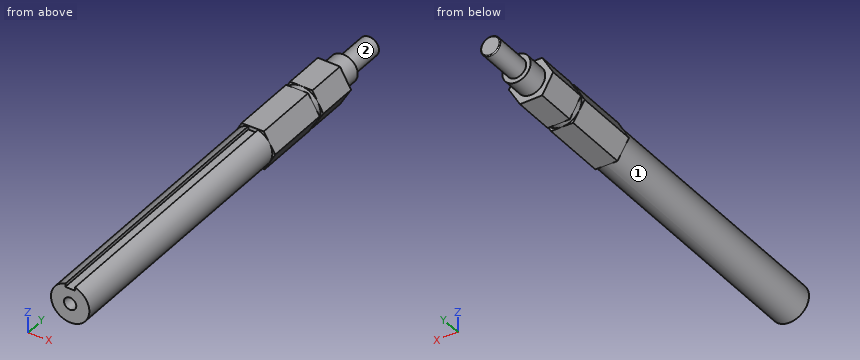
Autodesk Inventor part; units mm, degrees
ref_plane "YZ Plane" through (0, 0, 0) normal (1, 0, 0) x (0, 1, 0)
ref_plane "XZ Plane" through (0, 0, 0) normal (0, 1, 0) x (-1, 0, 0)
ref_plane "XY Plane" through (0, 0, 0) normal (0, 0, 1) x (1, 0, 0)
sketch "Sketch1" plane through (0, 0, 0) normal (0, 1, 0) x (-1, 0, 0)
  circle A0 centre (0, 0) radius 6.35
  dimension "d0" = 12.7
extrude "Extrusion1" add sketch "Sketch1" along normal mid plane 88.9
sketch "Sketch2" plane through (0, 44.45, 0) normal (0, 1, 0) x (1, 0, 0)
  circle A0 centre (0, 0) radius 6.35
  line L0 (3.8092, 6.2652) -> (7.3305, -0.1662)
  line L1 (7.3305, -0.1662) -> (3.5213, -6.4315)
  line L2 (3.5213, -6.4315) -> (-3.8092, -6.2652)
  line L3 (-3.8092, -6.2652) -> (-7.3305, 0.1662)
  line L4 (-7.3305, 0.1662) -> (-3.5213, 6.4315)
  line L5 (-3.5213, 6.4315) -> (3.8092, 6.2652)
  dimension "d4" = 12.7
extrude "Extrusion2" add sketch "Sketch2" along normal blind 21.59
sketch "Sketch3" plane through (0, 66.04, 0) normal (0, 1, 0) x (1, 0, 0)
  circle A0 centre (0, 0) radius 6.35
  dimension "d7" = 12.7
extrude "Extrusion3" add sketch "Sketch3" along normal blind 1.778
sketch "Sketch4" plane through (0, 67.818, 0) normal (0, 1, 0) x (1, 0, 0)
  circle A0 centre (0, 0) radius 6.35
  line L0 (7.3323, 0) -> (3.6662, -6.35)
  line L1 (3.6662, -6.35) -> (-3.6662, -6.35)
  line L2 (-3.6662, -6.35) -> (-7.3323, 0)
  line L3 (-7.3323, 0) -> (-3.6662, 6.35)
  line L4 (-3.6662, 6.35) -> (3.6662, 6.35)
  line L5 (3.6662, 6.35) -> (7.3323, 0)
  dimension "d10" = 12.7
extrude "Extrusion4" add sketch "Sketch4" along normal blind 13.462
sketch "Sketch5" plane through (0, 81.28, 0) normal (0, 1, 0) x (1, 0, 0)
  circle A0 centre (0, 0) radius 4.699
  dimension "d13" = 9.398
extrude "Extrusion5" add sketch "Sketch5" along normal blind 7.112
sketch "Sketch6" plane through (0, 88.392, 0) normal (0, 1, 0) x (1, 0, 0)
  circle A0 centre (0, 0) radius 4.699
  circle A1 centre (0, 0) radius 3.2258
  dimension "d16" = 6.4516
extrude "Extrusion6" add sketch "Sketch6" along normal blind 12.7 contours A1
fillet "Fillet1" radius 0.3175 1 edges at (-3.2258, 101.092, 0)
sketch "Sketch7" plane through (0, -44.45, 0) normal (0, -1, 0) x (1, 0, 0)
  line L0 (-1.5875, 6.8356) -> (1.5875, 6.8356)
  line L1 (1.5875, 6.8356) -> (1.5875, 5.0371)
  line L2 (1.5875, 5.0371) -> (-1.5875, 5.0371)
  line L3 (-1.5875, 5.0371) -> (-1.5875, 6.8356)
  line L4 (0, 11.7561) -> (0, 9.7432)
  line L5 (-3.323, -0.0429) -> (4.4977, -0.0429)
  dimension "d20" = 3.175
  dimension "d24" = 5.08
extrude "Extrusion7" cut sketch "Sketch7" against normal blind 88.9
sketch "Sketch8" plane through (0, -44.45, 0) normal (0, -1, 0) x (1, 0, 0)
  arc A0 (-1.5875, 6.1484) -> (1.5875, 6.1484) centre (0, 0) ccw
  circle A1 centre (0, 0) radius 2.032
  dimension "d27" = 4.064
extrude "Extrusion8" cut sketch "Sketch8" against normal blind 50.8
properties part number "Shaft"
The model under review builds one solid part; all positions refer to its coordinate system, in mm. Face numbers are marked on the shaded views. A direction names the side the tool comes from. Coordinates: 2 decimals unless noted, no trailing zeros. Write each loop counter-clockwise with the first axis right and the second up, starting at its lowest first coordinate (ties: lowest second). Pieces come first, ordered by that corner, then holes. Notation, with made-up numbers: M 83.25,-33 L 113.25,-33 A8 ccw 113.25,-24 Z; hole C -38,88.5 d6. An arc over 180 degrees is marked long. Put each result on its own line as item: value.
1) Wall thickness on probe 1 along Z at (x, y) = (0, -33); probe 2 along Y at (x, z) = (-1, -4.75); probe 3 along Z at (x, y) = (1.75, -34.5): over which ranges is each line inside the solid? List them lowest first. Write a range as [from, to].
Computed:
probe 1: z = [-6.35, -2.03], [2.03, 5.04]
probe 2: y = [-44.45, 81.28]
probe 3: z = [-6.1, -1.03], [1.03, 6.1]
2) Clearance check with flat-ended pins moving along their axes: pin 1 Ø3.5 at (x, y) = (0.5, 77) entering from -Z; pin 2 Ø6 at (x, y) = (2, 67) entering from -Z; pin 3 Ø3 at (y, z) = (-28, -4.5) entering from +X. State where each tip first meets the part, or that it passes through.
Computed:
pin 1: stops at z = -6.35
pin 2: stops at z = -6.37
pin 3: stops at x = 5.6
3) Add section B-B on y = 8.5. Give the boundary of the cut face in (x, z).
Computed:
outline: M -1.59,5.04 L -1.59,6.15 A6.35 ccw long 1.59,6.15 L 1.59,5.04 Z
4) For the marked faces 1 and 2, list the 3-axis set-ups (+Z, -Z, +X, -X, +Y, -Y) from which the entire face can be reached by the end or side of a thin tool; tool diameter is ignored.
Computed:
face 1: -Y
face 2: +Y
5) Add section A-A on y = 73. Give the boundary of the cut face in (x, z).
Computed:
outline: M -7.33,0 L -3.67,-6.35 L 3.67,-6.35 L 7.33,0 L 3.67,6.35 L -3.67,6.35 Z
